Here's how the part is built. I have some questions about the finished solid (model axes, mm). A direction names the side the tool comes from. Coordinates: 2 decimals unless noted, no trailing zeros. Write each loop counter-clockwise with the first axis right and the second up, starting at its lowest first coordinate (ties: lowest second). Pieces come first, ordered by that corner, then holes. Notation, with made-up numbers: (-27.5, 70) -> (15.5, 70) arc R10 cw to (15.5, 81) -> close; hole circle Ø4 at (85, -24). An arc over 180 degrees is marked (long way). Use a Markdown table: item, result. Add a question column.
Item 1: If we mould it in two halves opening along X, with no side actions, what happens to faces 1 (the flat face through (52, 30, 44)), 2 (the flat face through (34.3, 26.2, 45.6)), 3 (the flat face through (47, 26, 44))? For each: pulls with the +X half, pulls with the -X half, needs draft (parallel to the pull), parting line crosses it, or undercut.
Item 2: Imagine slicing it at A-A, the plane y = 12.5. Write out the boundary of the cut face in (x, z), and give its area (3 significant figures).
Item 3: Imagine slicing it at C-C, the plane z = 85. Count the separate pieces of the cut face and the enclosed holes in it, and give its area (3 significant figures).
Item 4: On a 3-axis mill with a long thin cutter (end or side, diameter ignored), from which of +Z, -Z, +X, -X, +Y, -Y can I reach the whole of each face in a straight line? I mean faces 4 (the flat face through (31.5, 13, 44)), 5 (the cylindrical face through (31.573, 26.487, 44.37)), 6 (the flat face through (-19, 26, 44)), 7 (the flat face through (42, 13, 44)), 8 (the flat face through (16, 29, 90)). Say none if no direction works.
Item 5: If I drill on line 1 along Z through (x, y) = (-33, 28.5); line 2 along X through (y, z) = (5.5, 11); line 3 along X through (y, z) = (14, 41), over which ranges is the centre line in solid material (lowest first)? Write a range as from..to.
Item 6: Imagine slicing it at B-B, the plane x = -33. Write out the boundary of the cut face in (y, z), and give its area (3 significant figures).
Item 7: Imagine slicing it at D-D, the plane y = 6.5. Write out the boundary of the cut face in (x, z).
Item 8: Will these pins go through, and if not, where does the flat tip stop? pin 1 Ø5 at (x, z) = (17, 37) entering from -Y; pin 2 Ø8 at (y, z) = (2.5, 59) entering from +X; pin 3 Ø10 at (x, z) = (-27.5, 80.5) entering from -Y.
```python
from build123d import *

# Parameters (mm, degrees)
F1_DEPTH     = 90
F2_R         = 3
F3_DEPTH     = 25
F4_W         = 3.5
F4_H         = 3.5
F5_DEPTH     = 300
F6_SIZE      = 3
F7_SIZE      = 3
F8_R         = 1
F9_T1_DEPTH  = 99.9215674165
F10_T1_DEPTH = 99.9215674165


# Not quite as in the source:
# - a fillet or chamfer that OpenCascade refuses, or shapes differently, is made with other operations: its cross-section is extruded or revolved along the edge and cut away or added


with BuildPart() as f1:
    # F0 (on Top) → F1 (new body)
    with BuildSketch(Plane.XY):
        Polygon((0, 26), (0, 0), (8, 0), (8, 10), (10.5, 10), (10.5, 16), (8, 16), (8, 26), (18, 26), (18, 23.5), (24, 23.5), (24, 26), (34, 26), (34, 16), (31.5, 16), (31.5, 10), (34, 10), (34, 0), (42, 0), (42, 26), (52, 26), (52, 34), (-38, 34), (-38, 26), align=None)
    extrude(amount=F1_DEPTH)

    # F2 (on face) → F3 (cut)
    with BuildSketch(Plane(origin=(0, 34, 0), x_dir=(-1, 0, 0), z_dir=(0, 1, 0))):
        with Locations((33, 85)):
            Circle(F2_R)
        with Locations((33, 5)):
            Circle(F2_R)
        with Locations((-47, 5)):
            Circle(F2_R)
        with Locations((-47, 85)):
            Circle(F2_R)
    extrude(amount=-F3_DEPTH, mode=Mode.SUBTRACT)

    # F4 (on face) → F5 (cut)
    with BuildSketch(Plane.XY.offset(90)):
        with Locations((8, 26)):
            Rectangle(F4_W, F4_H)
        with Locations((34, 26)):
            Rectangle(F4_W, F4_H)
    extrude(amount=-F5_DEPTH, mode=Mode.SUBTRACT)

    # F6
    f6_edges = [f1.edges().sort_by_distance(p)[0] for p in [
        (6.25, 27.75, 45),
    ]]
    chamfer(f6_edges, length=F6_SIZE)

    # F7
    f7_edges = [f1.edges().sort_by_distance(p)[0] for p in [
        (35.75, 27.75, 45),
    ]]
    chamfer(f7_edges, length=F7_SIZE)

    # F8
    f8_edges = [f1.edges().sort_by_distance(p)[0] for p in [
        (10.5, 10, 45),
        (10.5, 16, 45),
        (18, 23.5, 45),
        (24, 23.5, 45),
        (31.5, 10, 45),
        (31.5, 16, 45),
    ]]
    fillet(f8_edges, radius=F8_R)

    # F9: fillet of radius 2 on 2 edges, made by hand

    # F9_s2 → F9_t1 (cut)
    with BuildSketch(Plane.XY.offset(-4.9607837082)):
        with BuildLine():
            ThreePointArc((35.75, 24.25), (34.5, 23.5885621722), (34, 22.2656865167))
            Line((34, 22.2656865167), (34, 24.25))
            Line((34, 24.25), (35.75, 24.25))
        make_face()
        with BuildLine():
            ThreePointArc((30.2656865167, 26), (31.5885621722, 26.5), (32.25, 27.75))
            Line((32.25, 27.75), (32.25, 26))
            Line((32.25, 26), (30.2656865167, 26))
        make_face()
    extrude(amount=F9_T1_DEPTH, mode=Mode.SUBTRACT)

    # F10: fillet of radius 2 on 2 edges, made by hand

    # F10_s2 → F10_t1 (cut)
    with BuildSketch(Plane.XY.offset(-4.9607837082)):
        with BuildLine():
            ThreePointArc((11.7343134833, 26), (10.4114378278, 26.5), (9.75, 27.75))
            Line((9.75, 27.75), (9.75, 26))
            Line((9.75, 26), (11.7343134833, 26))
        make_face()
        with BuildLine():
            ThreePointArc((6.25, 24.25), (7.5, 23.5885621722), (8, 22.2656865167))
            Line((8, 22.2656865167), (8, 24.25))
            Line((8, 24.25), (6.25, 24.25))
        make_face()
    extrude(amount=F10_T1_DEPTH, mode=Mode.SUBTRACT)


solid = f1.part
```
Ans:
| question | item | result |
|---|---|---|
| 1 | face 1 | pulls with the +X half |
| 1 | face 2 | undercut |
| 1 | face 3 | needs draft |
| 2 | outline | (0, 0) -> (10.5, 0) -> (10.5, 90) -> (0, 90) -> close; (31.5, 0) -> (42, 0) -> (42, 90) -> (31.5, 90) -> close |
| 2 | area | 1,890 mm^2 |
| 3 | separate pieces | 3 |
| 3 | enclosed holes | 0 |
| 3 | area | 1,070 mm^2 |
| 4 | face 4 | +Z, -Z, -Y |
| 4 | face 5 | +Z, -Z |
| 4 | face 6 | +Z, -Z, -X, -Y |
| 4 | face 7 | +Z, -Z, +X, -Y |
| 4 | face 8 | +Z, +X, -X, +Y, -Y |
| 5 | line 1 | z = 0..2, 8..82, 88..90 |
| 5 | line 2 | x = 0..8, 34..42 |
| 5 | line 3 | x = 0..10.5, 31.5..42 |
| 6 | outline | (26, 0) -> (34, 0) -> (34, 2) -> (26, 2) -> close; (26, 8) -> (34, 8) -> (34, 82) -> (26, 82) -> close; (26, 88) -> (34, 88) -> (34, 90) -> (26, 90) -> close |
| 6 | area | 624 mm^2 |
| 7 | outline | (0, 0) -> (8, 0) -> (8, 90) -> (0, 90) -> close; (34, 0) -> (42, 0) -> (42, 90) -> (34, 90) -> close |
| 8 | pin 1 | stops at y = 23.5 |
| 8 | pin 2 | stops at x = 42 |
| 8 | pin 3 | stops at y = 26 |
